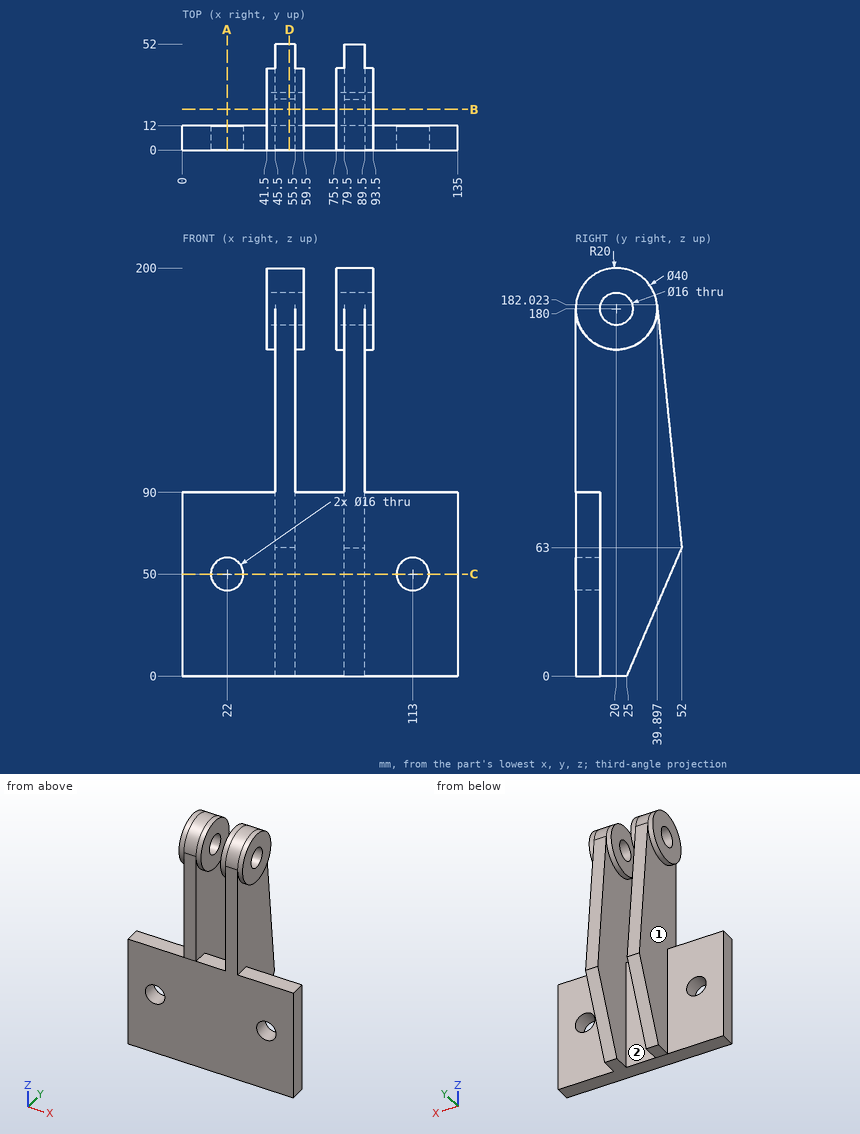
Input: dimensioned drawing with shaded views. Units: mm. Origin: part minimum x, y, z. Coordinates: 2 decimals unless noted, no trailing zeros. Order: outer loops, then holes, each group sorted by start corner. A loop starts at its lowest first (then second) coordinate and runs counter-clockwise, first axis right, second up. Notation, with made-up numbers: (66.5, 72) - (116.5, 72) arc R17 cw to (116.5, 90) - close; hole circle Ø3 at (-36.75, 60). An arc over 180 degrees is marked (long way). One line per item, written item: value.
1) Mould query, pull axis Z, two halves, no side actions, for the marked faces 1 and 2. Classes: released by +Z, released by -Z, zero draft, split by the parting line, or undercut.
Computed values:
face 1: undercut
face 2: zero draft
2) Cut plane A-A on x = 22. Output: boundary loops of the cut face in (y, z).
Computed values:
outline: (0, 0) - (12, 0) - (12, 42) - (0, 42) - close; (0, 58) - (12, 58) - (12, 90) - (0, 90) - close
3) Contact query for flat-ended pins moving along their axis: pin 1 (8 mm diameter, centred on y = 40.5, z = 55, fed in from -X); pin 2 (1 mm diameter, centred on x = 90.5, y = 33, fed in from -Z); pin 3 (12 mm diameter, centred on y = 14.5, z = 185.5, fed in from -X); pin 4 (9.5 mm diameter, centred on x = 22, z = 50, fed in from +Y). Output: stop coordinate, or through.
Computed values:
pin 1: stops at x = 45.5
pin 2: stops at z = 164.39
pin 3: stops at x = 41.5
pin 4: passes through
4) Cut plane D-D on x = 52.5. Output: boundary loops of the cut face in (y, z), plus the area to 3 significant figures.
Computed values:
outline: (0, 0) - (25, 0) - (52, 63) - (39.9, 182.02) arc R20 ccw to (0, 180) - close; hole circle Ø16 at (20, 180)
area: 8,240 mm^2
5) Cut plane C-C on z = 50. Output: boundary loops of the cut face in (x, y), plus the area to 3 significant figures.
Computed values:
outline: (0, 0) - (14, 0) - (14, 12) - (0, 12) - close; (30, 0) - (105, 0) - (105, 12) - (89.5, 12) - (89.5, 46.43) - (79.5, 46.43) - (79.5, 12) - (55.5, 12) - (55.5, 46.43) - (45.5, 46.43) - (45.5, 12) - (30, 12) - close; (121, 0) - (135, 0) - (135, 12) - (121, 12) - close
area: 1,920 mm^2
6) Cut plane B-B on y = 20. Output: boundary loops of the cut face in (x, z), plus the area to 3 significant figures.
Computed values:
outline: (41.5, 160) - (45.5, 160) - (45.5, 0) - (55.5, 0) - (55.5, 160) - (59.5, 160) - (59.5, 172) - (41.5, 172) - close; (41.5, 188) - (59.5, 188) - (59.5, 200) - (41.5, 200) - close; (75.5, 160) - (79.5, 160) - (79.5, 0) - (89.5, 0) - (89.5, 160) - (93.5, 160) - (93.5, 172) - (75.5, 172) - close; (75.5, 188) - (93.5, 188) - (93.5, 200) - (75.5, 200) - close
area: 4,060 mm^2
7) Ray query, line 1 (Y direction, x = 56, z = 180); line 2 (X direction, y = 12, z = 97); line 3 (Z direction, x = 22, y = 3.5). Return the intervals inside material, ascending. Write a range as [from, to].
Computed values:
line 1: y = [0, 12], [28, 40]
line 2: x = [45.5, 55.5], [79.5, 89.5]
line 3: z = [0, 42], [58, 90]
